```python
from build123d import *

# Parameters (mm, degrees)
SKETCH1_R           = 9
SKETCH1_R_2         = 1.05
BOSS_EXTRUDE1_DEPTH = 2
CHAMFER1_SIZE       = 4
CUT_EXTRUDE3_START  = -53
SKETCH6_R           = 1.05
CUT_EXTRUDE3_DEPTH  = 53
CUT_EXTRUDE4_START  = -2
SKETCH5_R           = 2.05
CUT_EXTRUDE4_DEPTH  = 53
CHAMFER2_SIZE       = 5
CHAMFER3_SIZE       = 5
CHAMFER3_SIZE_2     = 4.05977785
SKETCH8_W           = 40.645388092
SKETCH8_H           = 21.779978949
CUT_EXTRUDE5_DEPTH  = 34


with BuildPart() as part:
    # Sketch1 → Boss-Extrude1 (new body)
    with BuildSketch(Plane.XY):
        Circle(SKETCH1_R)
        with Locations((0, 6)):
            Circle(SKETCH1_R_2, mode=Mode.SUBTRACT)
        with Locations((-6, 0)):
            Circle(SKETCH1_R_2, mode=Mode.SUBTRACT)
        with Locations((0, -6)):
            Circle(SKETCH1_R_2, mode=Mode.SUBTRACT)
        with Locations((6, 0)):
            Circle(SKETCH1_R_2, mode=Mode.SUBTRACT)
    extrude(amount=BOSS_EXTRUDE1_DEPTH)

    # Sketch3 → Loft1 section 0
    with BuildSketch(Plane(origin=(0, 0, -50), x_dir=(-1, 0, 0), z_dir=(0, 0, -1))):
        with BuildLine():
            Line((-0.707106781, -16.970562748), (16.970562748, 0.707106781))
            Line((16.970562748, 0.707106781), (21.920310217, -4.242640687))
            Line((21.920310217, -4.242640687), (4.242640687, -21.920310217))
            Line((4.242640687, -21.920310217), (-0.707106781, -16.970562748))
        make_face()
    # Sketch2 → Loft1 section 1
    with BuildSketch(Plane(origin=(0, 0, 0), x_dir=(-1, 0, 0), z_dir=(0, 0, -1))):
        with BuildLine():
            Line((-15.202795796, -2.474873734), (2.474873734, 15.202795796))
            Line((2.474873734, 15.202795796), (15.202795796, 2.474873734))
            Line((15.202795796, 2.474873734), (-2.474873734, -15.202795796))
            Line((-2.474873734, -15.202795796), (-15.202795796, -2.474873734))
        make_face()
    loft()

    # Chamfer1
    # the kernel refuses this chamfer: 4 mm, written as the material it takes off along each edge
    with BuildSketch(Plane(origin=(-4.798944185, -22.476613715, 0), x_dir=(-0.7068394360706721, 0.7068394360706747, 0.027495876610586344), z_dir=(0.7071067811865488, 0.7071067811865462, 0))) as chamfer1_piece_1_section:
        Polygon((CHAMFER1_SIZE * 0.999621916911, -CHAMFER1_SIZE * 0.0274958766106), (-CHAMFER1_SIZE * 0.0274958766106, -CHAMFER1_SIZE * 0.999621916911), (0, 0), align=None)
    chamfer1_piece_1 = extrude(amount=38.573463904, mode=Mode.PRIVATE)
    chamfer1_piece_1 = chamfer1_piece_1 - Plane(origin=(0, 0, -1.322334287), x_dir=(1, 0, 0), z_dir=(0, 0, -1)) * Cylinder(9, 94, mode=Mode.PRIVATE)
    add(chamfer1_piece_1, mode=Mode.SUBTRACT)
    with BuildSketch(Plane(origin=(4.798944185, 22.476613715, 0), x_dir=(0.7068394360706721, -0.7068394360706749, 0.027495876610586396), z_dir=(-0.7071067811865489, -0.7071067811865461, 0))) as chamfer1_piece_2_section:
        Polygon((CHAMFER1_SIZE * 0.999621916911, -CHAMFER1_SIZE * 0.0274958766106), (-CHAMFER1_SIZE * 0.0274958766106, -CHAMFER1_SIZE * 0.999621916911), (0, 0), align=None)
    chamfer1_piece_2 = extrude(amount=38.573463904, mode=Mode.PRIVATE)
    chamfer1_piece_2 = chamfer1_piece_2 - Plane(origin=(0, 0, -1.322334287), x_dir=(1, 0, 0), z_dir=(0, 0, -1)) * Cylinder(9, 94, mode=Mode.PRIVATE)
    add(chamfer1_piece_2, mode=Mode.SUBTRACT)

    # Sketch6 → Cut-Extrude3 (cut)
    with BuildSketch(Plane.XY.offset(2).offset(CUT_EXTRUDE3_START)):
        with Locations(Location((0, -6, 0), (0, 0, 45))):
            Circle(SKETCH6_R)
        with Locations(Location((6, 0, 0), (0, 0, 45))):
            Circle(SKETCH6_R)
        with Locations(Location((0, 6, 0), (0, 0, 45))):
            Circle(SKETCH6_R)
        with Locations(Location((-6, 0, 0), (0, 0, 45))):
            Circle(SKETCH6_R)
    extrude(amount=CUT_EXTRUDE3_DEPTH, mode=Mode.SUBTRACT)

    # Sketch5 → Cut-Extrude4 (cut)
    with BuildSketch(Plane.XY.offset(2).offset(CUT_EXTRUDE4_START)):
        with Locations(Location((-6, 0, 0), (0, 0, 45))):
            Circle(SKETCH5_R)
        with Locations(Location((0, -6, 0), (0, 0, 45))):
            Circle(SKETCH5_R)
        with Locations(Location((0, 6, 0), (0, 0, 45))):
            Circle(SKETCH5_R)
        with Locations(Location((6, 0, 0), (0, 0, 45))):
            Circle(SKETCH5_R)
    extrude(amount=-CUT_EXTRUDE4_DEPTH, mode=Mode.SUBTRACT)

    # Chamfer2
    chamfer2_edges = [part.edges().sort_by_distance(p)[0] for p in [
        (-10.302545802, 7.375123728, -27),
        (7.375123728, -10.302545802, -27),
    ]]
    chamfer(chamfer2_edges, length=CHAMFER2_SIZE)

    # Chamfer3
    # the kernel refuses this chamfer: 5, 4.05977785 mm, written as the material it takes off along each edge
    with BuildSketch(Plane(origin=(13.909394742, 12.166115274, 0), x_dir=(0.009375164320641791, -0.2414717461398742, -0.9703625621952453), z_dir=(-0.9992471568778876, -0.03879586925767199, 0))) as chamfer3_piece_1_section:
        Polygon((CHAMFER3_SIZE * 0.999621916911, CHAMFER3_SIZE * 0.0274958766106), (CHAMFER3_SIZE_2 * 0.241653673437, CHAMFER3_SIZE_2 * 0.970362562158), (0, 0), align=None)
    chamfer3_piece_1 = extrude(amount=27.189276823, mode=Mode.PRIVATE)
    chamfer3_piece_1 = chamfer3_piece_1 - Plane(origin=(0, 0, -1.642174888), x_dir=(1, 0, 0), z_dir=(0, 0, -1)) * Cylinder(9, 75, mode=Mode.PRIVATE)
    add(chamfer3_piece_1, mode=Mode.SUBTRACT)
    with BuildSketch(Plane(origin=(12.166115274, 13.909394742, 0), x_dir=(-0.2414717461398332, 0.009375164320638266, -0.9703625621952554), z_dir=(-0.03879586925766401, -0.9992471568778879, 0))) as chamfer3_piece_2_section:
        Polygon((CHAMFER3_SIZE * 0.999621916911, -CHAMFER3_SIZE * 0.0274958766106), (CHAMFER3_SIZE_2 * 0.241653673437, -CHAMFER3_SIZE_2 * 0.970362562158), (0, 0), align=None)
    chamfer3_piece_2 = extrude(amount=27.189276823, mode=Mode.PRIVATE)
    chamfer3_piece_2 = chamfer3_piece_2 - Plane(origin=(0, 0, -1.642174892), x_dir=(1, 0, 0), z_dir=(0, 0, -1)) * Cylinder(9, 75, mode=Mode.PRIVATE)
    add(chamfer3_piece_2, mode=Mode.SUBTRACT)

    # Sketch8 → Cut-Extrude5 (cut)
    with BuildSketch(Plane(origin=(-8.838834765, 8.838834765, 0), x_dir=(0, 0, 1), z_dir=(-0.7071067811865461, 0.7071067811865489, 0))):
        with Locations((-29.677305954, -22.389989475)):
            Rectangle(SKETCH8_W, SKETCH8_H)
    extrude(amount=-CUT_EXTRUDE5_DEPTH, mode=Mode.SUBTRACT)


solid = part.part
```
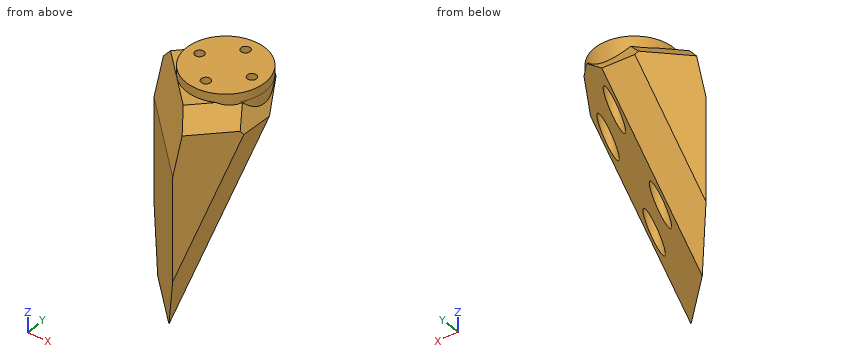
CAD build for the part. Positions are in the model's coordinates, mm. Round coordinates to 2 decimals unless told otherwise and drop trailing zeros. Answer as CSV lines item,"result". Start each with the question number.
1. Pin check, flat tips, straight feed: pin 1 (4 mm diameter, centred on y = -12.5, z = -18, fed in from +X); pin 2 (6.5 mm diameter, centred on x = 6, y = 0, fed in from -Z); pin 3 (1 mm diameter, centred on y = -5.5, z = -37, fed in from -X). Stop position of each tip, or through.
2. Saw through at A-A, the plane z = -1.5. Count the separate pieces of the cut face and the enclosed holes in it, and give its area (3 significant figures).
3. Drill centre lines: L1, parallel to Y at x = 0, z = 0.7; L2, parallel to Y at x = 0, z = -6.25; L3, parallel to Y at x = -6.5, z = -15. Where is each one in solid material? Low to high. Write a range as [from, to].
Model answer:
1,pin 1,"stops at x = 6.58"
1,pin 2,"stops at z = -19.53"
1,pin 3,"stops at x = -11.26"
2,separate pieces,"1"
2,enclosed holes,"4"
2,area,"263 mm²"
3,L1,"y = [-9, -7.05], [-4.95, 4.95], [7.05, 9]"
3,L2,"y = [-14.41, -8.05], [-3.95, 3.95], [8.05, 9.1]"
3,L3,"y = [-9.76, -1.99], [1.99, 7.19]"
